The listing builds one solid part. Answer for the finished solid, in the listing's coordinates (mm). A direction names the side the tool comes from. Coordinates: 2 decimals unless noted, no trailing zeros. Order: outer loops, then holes, each group sorted by start corner. A loop starts at its lowest first (then second) coordinate and runs counter-clockwise, first axis right, second up. Notation, with made-up numbers: (60.25, -18.75) -> (77.25, -18.75) arc R23 cw to (77.25, 16.25) -> close; hole circle Ø9 at (-23, -18.75). An arc over 180 degrees is marked (long way). Answer in a Markdown table with one row per item. Add a question column.
```python
from build123d import *

# Parameters (mm, degrees)
SERVO_SHELF_START           = -36.480025
SKETCH1_W                   = 48
SKETCH1_H                   = 38
SKETCH1_W_2                 = 13
SKETCH1_H_2                 = 24.35
SERVO_SHELF_DEPTH           = 3
OUTBOARD_RISER_START        = -34.480025
SKETCH2_W                   = 6
SKETCH2_H                   = 14
OUTBOARD_RISER_DEPTH        = 33.480025
PLATE_ATTACHMENT_FOOT_START = -2
SKETCH3_W                   = 20
SKETCH3_H                   = 14
PLATE_ATTACHMENT_FOOT_DEPTH = 2


with BuildPart() as part:
    # Sketch1 → Servo_Shelf (new body)
    with BuildSketch(Plane.XY.offset(SERVO_SHELF_START)):
        with Locations((-46, 19)):
            Rectangle(SKETCH1_W, SKETCH1_H)
        with Locations((-60, 18.825)):
            Rectangle(SKETCH1_W_2, SKETCH1_H_2, mode=Mode.SUBTRACT)
    extrude(amount=SERVO_SHELF_DEPTH)

    # Sketch2 → Outboard_Riser (add)
    with BuildSketch(Plane.XY.offset(OUTBOARD_RISER_START)):
        with Locations((-37, 21)):
            Rectangle(SKETCH2_W, SKETCH2_H)
    extrude(amount=OUTBOARD_RISER_DEPTH)

    # Sketch3 → Plate_Attachment_Foot (add)
    with BuildSketch(Plane.XY.offset(PLATE_ATTACHMENT_FOOT_START)):
        with Locations((-30, 21)):
            Rectangle(SKETCH3_W, SKETCH3_H)
    extrude(amount=PLATE_ATTACHMENT_FOOT_DEPTH)


solid = part.part
```
Q1. For faces 1 (the face through (-22, 19, -35)), 2 (the face through (-60, 6.65, -35)), 3 (the face through (-35, 14, -14)), 4 (the face through (-34, 21, -18)), determine the directions among +Z, -Z, +X, -X, +Y, -Y from which every point of the face is accessible in a straight line to the end or side of a thin tool.
Q2. Straight lines are drawn through the part: line 1 (Z direction, x = -32, y = 23); line 2 (X direction, y = 22.5, z = -17); line 3 (Z direction, x = -45, y = 30). For each, find the intervals that lie inside material, in ascending order.
Q3. Determine the mould class of faces 5 (the face through (-46, 0, -35)), 6 (the face through (-60, 31, -35)), 7 (the face through (-20, 21, -1)) for opening direction X: +X half, -X half, draft (parallel to the pull), parting line (faces both ways), or undercut.
Q4. A cutting plane is placed at A-A (x = -31). Determine the outline of the cut face in (y, z), then the cut area to 3 significant figures.
Q5. A cutting plane is placed at D-D (z = -26). Determine the outline of the cut face in (x, y), then the cut area to 3 significant figures.
Q6. Given pin 1 (6 mm diameter, centred on x = -54, y = 25.5, fed in from +Z); pin 2 (3.5 mm diameter, centred on y = 20.5, z = -34.5, fed in from +X); pin 3 (1.5 mm diameter, centred on y = 19, z = -29, fed in from -X), each flat-ended and moving along its own axis, determine where each tip first touches the part or whether it passes through.
Q7. A cutting plane is placed at C-C (y = 32.5). Determine the outline of the cut face in (x, z).
Q8. A cutting plane is placed at B-B (x = -36.5). Determine the outline of the cut face in (y, z), then the cut area to 3 significant figures.
Returned:
| question | item | result |
|---|---|---|
| 1 | face 1 | -Z, +X, +Y, -Y |
| 1 | face 2 | +Z, -Z |
| 1 | face 3 | +Z, +X, -X, -Y |
| 1 | face 4 | +X, +Y, -Y |
| 2 | line 1 | z = -36.48 to -33.48, -2 to 0 |
| 2 | line 2 | x = -40 to -34 |
| 2 | line 3 | z = -36.48 to -33.48 |
| 3 | face 5 | draft |
| 3 | face 6 | undercut |
| 3 | face 7 | +X half |
| 4 | outline | (0, -36.48) -> (38, -36.48) -> (38, -33.48) -> (0, -33.48) -> close; (14, -2) -> (28, -2) -> (28, 0) -> (14, 0) -> close |
| 4 | area | 142 mm² |
| 5 | outline | (-40, 14) -> (-34, 14) -> (-34, 28) -> (-40, 28) -> close |
| 5 | area | 84.0 mm² |
| 6 | pin 1 | stops at z = -33.48 |
| 6 | pin 2 | stops at x = -22 |
| 6 | pin 3 | stops at x = -40 |
| 7 | outline | (-70, -36.48) -> (-22, -36.48) -> (-22, -33.48) -> (-70, -33.48) -> close |
| 8 | outline | (0, -36.48) -> (38, -36.48) -> (38, -33.48) -> (28, -33.48) -> (28, 0) -> (14, 0) -> (14, -33.48) -> (0, -33.48) -> close |
| 8 | area | 583 mm² |
